Geometry check sheet. Reference: the model listing, model coordinates, mm. Give positions to 0.01 mm unless a question says otherwise; leave off trailing zeros. Write each loop counter-clockwise with the first axis right and the second up, starting at its lowest first coordinate (ties: lowest second). Pieces come first, ordered by that corner, then holes. Notation, with made-up numbers: M 82,-20 L 123,-20 A15 cw 123,-10 Z; hole C -17.75,42.25 d2. An arc over 180 degrees is marked long. Write each question's results on one line, items separated by ' | '.
```python
from build123d import *

# Parameters (mm, degrees)
RESSALTO_EXTRUS_O1_DEPTH = 2


with BuildPart() as part:
    # Model → Ressalto-extrusão1 (new body)
    with BuildSketch(Plane.XY):
        with BuildLine():
            Line((-58.8502, -89.6424), (-58.8502, -94.0776))
            add(Edge.make_bspline(
                [(-58.8502, -94.0776), (-9.0376, -97.7844), (-12.8956, -128.2849), (-58.8502, -128.9929)],
                knots=[0.047619048, 0.047619048, 0.047619048, 0.047619048, 0.095238095, 0.095238095, 0.095238095, 0.095238095], degree=3))
            Line((-58.8502, -128.9929), (-58.8502, -134.309))
            Line((-58.8502, -134.309), (-3.1835, -134.309))
            Line((-3.1835, -134.309), (-3.1835, -110.4605))
            Line((-3.1835, -110.4605), (-1.1835, -110.4605))
            Line((-1.1835, -110.4605), (-1.1835, -134.309))
            Line((-1.1835, -134.309), (54.4831, -134.309))
            Line((54.4831, -134.309), (54.4831, -128.9929))
            add(Edge.make_bspline(
                [(54.4831, -128.9929), (8.5266, -128.2849), (4.6696, -97.7845), (54.4831, -94.0776)],
                knots=[0.428571429, 0.428571429, 0.428571429, 0.428571429, 0.476190476, 0.476190476, 0.476190476, 0.476190476], degree=3))
            Line((54.4831, -94.0776), (54.4831, -89.6424))
            Line((54.4831, -89.6424), (26.1498, -89.6424))
            Line((26.1498, -89.6424), (26.1498, -87.6372))
            Line((26.1498, -87.6372), (19.4831, -87.6372))
            Line((19.4831, -87.6372), (19.4831, -89.6424))
            Line((19.4831, -89.6424), (-23.8502, -89.6424))
            Line((-23.8502, -89.6424), (-23.8502, -87.6372))
            Line((-23.8502, -87.6372), (-30.5169, -87.6372))
            Line((-30.5169, -87.6372), (-30.5169, -89.6424))
            Line((-30.5169, -89.6424), (-58.8502, -89.6424))
        make_face()
    extrude(amount=RESSALTO_EXTRUS_O1_DEPTH)


solid = part.part
```
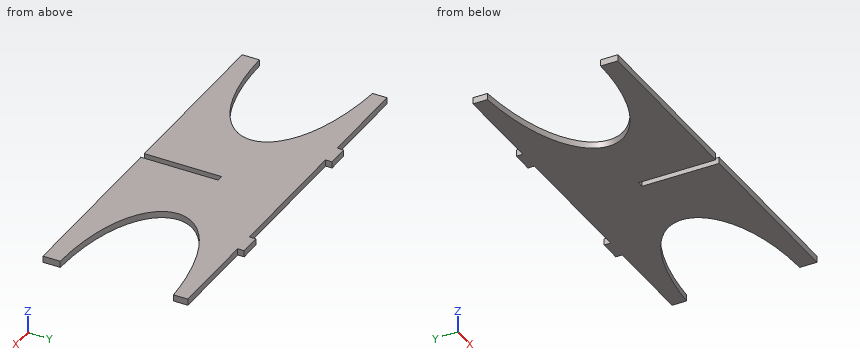
Q1. Material ranges on probe 1 along X at (y, z) = (-112.5, 0.5); probe 2 along X at (y, z) = (-129.5, 1.55); probe 3 along Y at (x, z) = (-42.5, 0.35), recorded low to high. Write a range as [from, to].
Answer key:
probe 1: x = [-22.93, -3.18], [-1.18, 18.56] | probe 2: x = [-58.85, -3.18], [-1.18, 54.48] | probe 3: y = [-134.31, -127.2], [-96.66, -89.64]
Q2. Section check A-A (x = 17). Enter the section's corners in (y, z).
Answer key:
outline: M -134.31,0 L -89.64,0 L -89.64,2 L -134.31,2 Z
Q3. Depth check by flat-ended pin: P1, Ø1, axis at y = -107.5, z = 0.5, coming from the +X side; P2, Ø1, axis at x = -48.5, z = 1, coming from the +Y side; P3, Ø3, axis at x = 38, y = -127.5, coming from the -Z side; P4, Ø1, axis at x = -2, z = 1.5, coming from the -Y side. Enter the tip coordinate at first touch or a pass-through.
Answer key:
P1: stops at x = 20.18 | P2: stops at y = -89.64 | P3: stops at z = 0 | P4: stops at y = -110.46
